from build123d import *

# Parameters (mm, degrees)
F1_DEPTH  = 20
F2_R      = 10
F3_R      = 6.35
F4_DEPTH  = 80.001
F6_D      = 5.4102
F6_DEPTH  = 12
F6_TIP    = 1.6253880605
F7_R      = 5
F8_DEPTH  = 50.001
F9_R      = 2.5
F10_DEPTH = 5
F11_R     = 0.5
F12_R     = 15


with BuildPart() as f1:
    # F0 (on Front) → F1 (new body, symmetric)
    with BuildSketch(Plane.XZ):
        Polygon((0, 80), (0, 0), (50, 0), (50, 12), (6, 12), (6, 80), align=None)
    extrude(amount=F1_DEPTH, both=True)

    # F2
    f2_edges = [f1.edges().sort_by_distance(p)[0] for p in [
        (6, 0, 12),
    ]]
    fillet(f2_edges, radius=F2_R)

    # F3 (on face) → F4 (cut, through all)
    with BuildSketch(Plane(origin=(0, 0, 0), x_dir=(1, 0, 0), z_dir=(0, 0, -1))):
        with Locations((35, 0)):
            Circle(F3_R)
    extrude(amount=-F4_DEPTH, mode=Mode.SUBTRACT)

    # F6
    with Locations(Plane(origin=(0, 0, 0), x_dir=(0, -1, 0), z_dir=(-1, 0, 0))):
        with Locations((0, 6)):
            Hole(F6_D / 2, depth=F6_DEPTH)
            with Locations((0, 0, -(F6_DEPTH + F6_TIP / 2))):  # 118° drill point
                Cone(0, F6_D / 2, F6_TIP, mode=Mode.SUBTRACT)

    # F7 (on face) → F8 (cut, through all)
    with BuildSketch(Plane(origin=(0, 0, 0), x_dir=(0, -1, 0), z_dir=(-1, 0, 0))):
        with BuildLine():
            ThreePointArc((-20, 76), (-10.1980390272, 78.9901951359), (0, 80))
            Line((0, 80), (-20, 80))
            Line((-20, 80), (-20, 76))
        make_face()
        with BuildLine():
            ThreePointArc((0, 80), (10.1980390272, 78.9901951359), (20, 76))
            Line((20, 76), (20, 80))
            Line((20, 80), (0, 80))
        make_face()
        with Locations((0, 70)):
            Circle(F7_R)
    extrude(amount=-F8_DEPTH, mode=Mode.SUBTRACT)

    # F9 (on face) → F10 (join)
    with BuildSketch(Plane(origin=(0, 0, 0), x_dir=(0, -1, 0), z_dir=(-1, 0, 0))):
        with Locations((0, 40)):
            Circle(F9_R)
    extrude(amount=F10_DEPTH)

    # F11
    f11_edges = [f1.edges().sort_by_distance(p)[0] for p in [
        (0, 2.5, 40),
        (-5, 2.5, 40),
    ]]
    fillet(f11_edges, radius=F11_R)

    # F12
    f12_edges = [f1.edges().sort_by_distance(p)[0] for p in [
        (50, -20, 6),
        (50, 20, 6),
    ]]
    fillet(f12_edges, radius=F12_R)


solid = f1.part
The listing builds one solid part. Answer for the finished solid, in the listing's coordinates (mm). A direction names the side the tool comes from. Coordinates: 2 decimals unless noted, no trailing zeros. Write each loop counter-clockwise with the first axis right and the second up, starting at its lowest first coordinate (ties: lowest second). Pieces come first, ordered by that corner, then holes. Notation, with made-up numbers: M 20,44 L 45,44 A20 ccw 45,77 Z; hole C 31.25,22 d1. An arc over 180 degrees is marked long. Use one line per item in the form item = value.
Item 1: Find section D-D, the plane y = 12. Give the vertices of the cut face in (x, z), plus the area to 3 significant figures.
Model answer:
outline = M 0,0 L 48.27,0 L 48.27,12 L 16,12 A10 cw 6,22 L 6,78.6 L 0,78.6 Z
area = 1,000 mm2
Item 2: For faces 5 (the face through (25, 0, 0)), 6 (the face through (6.08, -0.59, 3.36)), 7 (the face through (29, -5, 12)), determine the directions among +Z, -Z, +X, -X, +Y, -Y from which every point of the face is accessible in a straight line to the end or side of a thin tool.
Model answer:
face_5 = -Z, +X, -X, +Y, -Y
face_6 = -X
face_7 = +Z, +X, +Y, -Y
Item 3: Find the intervals of material crossed by probe 1 along Y at (x, z) = (8.25, 6); probe 2 along Y at (x, z) = (35, 5.25); probe 3 along X at (y, z) = (0, 6), in increasing order.
Model answer:
probe_1 = -20 to -2.71, 2.71 to 20
probe_2 = -20 to -6.35, 6.35 to 20
probe_3 = 13.63 to 28.65, 41.35 to 50
Item 4: Given P1, Ø10, axis at x = 27.5, z = 16, coming from the +Y side; P2, Ø2, axis at y = -12.5, z = 33, coming from the +X side; P3, Ø5, axis at y = 0, z = 6, coming from the -X side; P4, Ø9, axis at y = 0, z = 70, coming from the +X side, each flat-ended and moving along its own axis, determine where each tip first touches the part or whether it passes through.
Model answer:
P1 = 20
P2 = 6
P3 = 12.12
P4 = through
Item 5: Find section A-A, the plane z = 40. Give the vertices of the cut face in (x, y).
Model answer:
outline = M -5,-2 A0.5 ccw -4.5,-2.5 L -0.5,-2.5 A0.5 cw 0,-3 L 0,-20 L 6,-20 L 6,20 L 0,20 L 0,3 A0.5 cw -0.5,2.5 L -4.5,2.5 A0.5 ccw -5,2 Z
Item 6: Find section B-B, the plane y = -17. Give the vertices of the cut face in (x, z).
Model answer:
outline = M 0,0 L 44,0 L 44,12 L 16,12 A10 cw 6,22 L 6,77.14 L 0,77.14 Z
Item 7: The mould has two halves that part along Y. Classify faces 1 (the face through (2.96, 1.08, 65.12)), 2 (the face through (6, 0, 51)), 3 (the face through (-2.47, 0.54, 37.56)), 4 (the face through (5.8, 20, 26.9)): released by +Y, released by -Y, zero draft, split by the parting line, or undercut.
Model answer:
face_1 = undercut
face_2 = zero draft
face_3 = split by the parting line
face_4 = released by +Y
Item 8: Find section C-C, the plane x = 8.5. Give the vertices of the cut face in (y, z).
Model answer:
outline = M -20,0 L 20,0 L 20,15.39 L -20,15.39 Z; hole C 0,6 d5.41
